```python
from build123d import *

# Parameters (mm, degrees)
BOSS_EXTRUDE1_DEPTH = 34
SKETCH2_R           = 11
BOSS_EXTRUDE2_DEPTH = 2
SKETCH3_R           = 2.5
BOSS_EXTRUDE3_DEPTH = 24
SKETCH8_W           = 16.3
SKETCH8_H           = 10
BOSS_EXTRUDE4_DEPTH = 7.3


# Read off the part's stored shape, not the designer's step: M3 Tapped Hole1
with BuildPart() as part:
    # Sketch1 → Boss-Extrude1 (new body)
    with BuildSketch(Plane(origin=(0, 0, 0), x_dir=(1, 0, 0), z_dir=(0, 1, 0))):
        Polygon((-17.033766184, 21.15), (17.033766184, 21.15), (21.15, 17.033766184), (21.15, -17.033766184), (17.033766184, -21.15), (-17.033766184, -21.15), (-21.15, -17.033766184), (-21.15, 17.033766184), align=None)
    extrude(amount=BOSS_EXTRUDE1_DEPTH)

    # Sketch2 → Boss-Extrude2 (add)
    with BuildSketch(Plane(origin=(0, 34, 0), x_dir=(1, 0, 0), z_dir=(0, 1, 0))):
        with Locations(Location((0, 0, 0), (0, 0, 270))):
            Circle(SKETCH2_R)
    extrude(amount=BOSS_EXTRUDE2_DEPTH)

    # Sketch3 → Boss-Extrude3 (add)
    with BuildSketch(Plane(origin=(0, 34, 0), x_dir=(1, 0, 0), z_dir=(0, 1, 0))):
        with Locations(Location((0, 0, 0), (0, 0, 270))):
            Circle(SKETCH3_R)
    extrude(amount=BOSS_EXTRUDE3_DEPTH)

    # M3 Tapped Hole1 outline → M3 Tapped Hole1 (revolve, cut)
    with BuildSketch(Plane(origin=(15.5, 0, -15.5), x_dir=(1, 0, 0), z_dir=(0, 0, 1))):
        Polygon((0, 34), (0, 28.748924226), (1.25, 29.5), (1.25, 34), align=None)
    revolve(axis=Axis((15.5, 0, -15.5), (0, 1, 0)), mode=Mode.SUBTRACT)

    # M3 Tapped Hole1 2 outline → M3 Tapped Hole1 2 (revolve, cut)
    with BuildSketch(Plane(origin=(-15.5, 0, 15.5), x_dir=(1, 0, 0), z_dir=(0, 0, 1))):
        Polygon((0, 34), (0, 28.748924226), (1.25, 29.5), (1.25, 34), align=None)
    revolve(axis=Axis((-15.5, 0, 15.5), (0, 1, 0)), mode=Mode.SUBTRACT)

    # M3 Tapped Hole1 3 outline → M3 Tapped Hole1 3 (revolve, cut)
    with BuildSketch(Plane(origin=(15.5, 0, 15.5), x_dir=(1, 0, 0), z_dir=(0, 0, 1))):
        Polygon((0, 34), (0, 28.748924226), (1.25, 29.5), (1.25, 34), align=None)
    revolve(axis=Axis((15.5, 0, 15.5), (0, 1, 0)), mode=Mode.SUBTRACT)

    # M3 Tapped Hole1 4 outline → M3 Tapped Hole1 4 (revolve, cut)
    with BuildSketch(Plane(origin=(-15.5, 0, -15.5), x_dir=(1, 0, 0), z_dir=(0, 0, 1))):
        Polygon((0, 34), (0, 28.748924226), (1.25, 29.5), (1.25, 34), align=None)
    revolve(axis=Axis((-15.5, 0, -15.5), (0, 1, 0)), mode=Mode.SUBTRACT)

    # Sketch8 → Boss-Extrude4 (add)
    with BuildSketch(Plane.XY.offset(21.15)):
        with Locations((0, 5)):
            Rectangle(SKETCH8_W, SKETCH8_H)
    extrude(amount=BOSS_EXTRUDE4_DEPTH)


solid = part.part
```
Verification items for the finished model (mm, model axes). A direction names the side the tool comes from. Give positions to 0.01 mm unless a question says otherwise; leave off trailing zeros. Order: outer loops, then holes, each group sorted by start corner. A loop starts at its lowest first (then second) coordinate and runs counter-clockwise, first axis right, second up. Notation, with made-up numbers: (-32.75, -9.75) -> (-1.75, -9.75) arc R11 ccw to (-1.75, 7.25) -> close; hole circle Ø7 at (63.25, 35). An arc over 180 degrees is marked (long way). Use a Markdown table: item, result.
1) Section check C-C, the plane z = 0. Record the boundary of the cut face in (x, y), then the cut area to 3 significant figures.
Results:
| item | result |
|---|---|
| outline | (-21.15, 0) -> (21.15, 0) -> (21.15, 34) -> (11, 34) -> (11, 36) -> (2.5, 36) -> (2.5, 58) -> (-2.5, 58) -> (-2.5, 36) -> (-11, 36) -> (-11, 34) -> (-21.15, 34) -> close |
| area | 1,590 mm² |
2) Section check D-D, the plane y = 24.5. Record the boundary of the cut face in (x, z), then the cut area to 3 significant figures.
Results:
| item | result |
|---|---|
| outline | (-21.15, -17.03) -> (-17.03, -21.15) -> (17.03, -21.15) -> (21.15, -17.03) -> (21.15, 17.03) -> (17.03, 21.15) -> (-17.03, 21.15) -> (-21.15, 17.03) -> close |
| area | 1,760 mm² |
3) Tool access check on faces 1 (the cylindrical face through (-16.421, 31.782, -16.345)), 2 (the flat face through (0, 0, 3)), 3 (the flat face through (-19.121, 16.762, -19.063)), 4 (the flat face through (0, 10, 25)), 5 (the flat face through (8.15, 5, 25)). Record the directions out of +Z, -Z, +X, -X, +Y, -Y that give a thin tool (end or side, any length) a straight path to the whole face; none if there is none.
Results:
| item | result |
|---|---|
| face 1 | +Y |
| face 2 | +Z, -Z, +X, -X, -Y |
| face 3 | -Z, -X, +Y, -Y |
| face 4 | +Z, +X, -X, +Y |
| face 5 | +Z, +X, +Y, -Y |
4) Depth check by flat-ended pin: pin 1 Ø1.5 at (x, z) = (15, 20) entering from +Y; pin 2 Ø1.5 at (x, y) = (0, 19) entering from +Z; pin 3 Ø8 at (y, z) = (7, 24.5) entering from -X. Enter the tip coordinate at first touch or a pass-through.
Results:
| item | result |
|---|---|
| pin 1 | y = 34 |
| pin 2 | z = 21.15 |
| pin 3 | x = -17.68 |
5) Material ranges on probe 1 along Z at (x, y) = (15.5, 32.3); probe 2 along X at (y, z) = (30, 15), recorded low to high.
Results:
| item | result |
|---|---|
| probe 1 | -21.15 to -16.75, -14.25 to 14.25, 16.75 to 21.15 |
| probe 2 | -21.15 to -16.65, -14.35 to 14.35, 16.65 to 21.15 |
6) Section check A-A, the plane y = 5. Record the boundary of the cut face in (x, z), then the cut area to 3 significant figures.
Results:
| item | result |
|---|---|
| outline | (-21.15, -17.03) -> (-17.03, -21.15) -> (17.03, -21.15) -> (21.15, -17.03) -> (21.15, 17.03) -> (17.03, 21.15) -> (8.15, 21.15) -> (8.15, 28.45) -> (-8.15, 28.45) -> (-8.15, 21.15) -> (-17.03, 21.15) -> (-21.15, 17.03) -> close |
| area | 1,870 mm² |
7) Section check B-B, the plane x = 0. Record the boundary of the cut face in (y, z).
Results:
| item | result |
|---|---|
| outline | (0, -21.15) -> (34, -21.15) -> (34, -11) -> (36, -11) -> (36, -2.5) -> (58, -2.5) -> (58, 2.5) -> (36, 2.5) -> (36, 11) -> (34, 11) -> (34, 21.15) -> (10, 21.15) -> (10, 28.45) -> (0, 28.45) -> close |
8) Mould release check, pull along X, two halves, no side actions. Record for faces 6 (the flat face through (19.063, 16.762, -19.121)), 7 (the conical face through (15.45, 28.88, 15.71)), 8 (the flat face through (0, 36, -3)): pulls with the +X half, pulls with the -X half, needs draft (parallel to the pull), parting line crosses it, or undercut.
Results:
| item | result |
|---|---|
| face 6 | pulls with the +X half |
| face 7 | undercut |
| face 8 | needs draft |
